```python
from build123d import *

# Parameters (mm, degrees)
BOSS_EXTRUDE4_DEPTH  = 1.5875
M3_CLEARANCE_HOLE3_D = 3
M3_CLEARANCE_HOLE1_D = 3.1
M3_CLEARANCE_HOLE4_D = 2.95
M3_CLEARANCE_HOLE2_D = 3.1
M3_CLEARANCE_HOLE5_D = 3
BOSS_EXTRUDE6_DEPTH  = 3.175
FILLET1_R            = 2
FILLET3_R            = 1


with BuildPart() as part:
    # Sketch1 → Boss-Extrude4 (new, symmetric)
    with BuildSketch(Plane(origin=(0, 0, 0), x_dir=(1, 0, 0), z_dir=(0, 1, 0))):
        with BuildLine():
            Line((-62.799553621, 32.496136604), (-73.969425011, 32.691107434))
            Line((-73.969425011, 32.691107434), (-77.053684287, 35.88495141))
            ThreePointArc((-77.053684287, 35.88495141), (-84.36642289, 10.358894189), (-83.446216027, -16.178041625))
            Line((-83.446216027, -16.178041625), (-79.680911643, -13.825218315))
            Line((-79.680911643, -13.825218315), (-69.484649137, -16.179210996))
            Line((-69.484649137, -16.179210996), (-43.894490772, -57.132025032))
            Line((-43.894490772, -57.132025032), (-43.894490772, -64.826600275))
            Line((-43.894490772, -64.826600275), (-43.094490772, -64.826600275))
            Line((-43.094490772, -64.826600275), (-34, -64.826600275))
            Line((-34, -64.826600275), (-34, -55.55))
            Line((-34, -55.55), (-34, -53.55))
            Line((-34, -53.55), (-20, -53.55))
            Line((-20, -53.55), (-19.718918331, -55.55))
            Line((-19.718918331, -55.55), (19.718918331, -55.55))
            Line((19.718918331, -55.55), (20, -53.55))
            Line((20, -53.55), (34, -53.55))
            Line((34, -53.55), (34, -55.55))
            Line((34, -55.55), (34, -64.826600275))
            Line((34, -64.826600275), (43.094490772, -64.826600275))
            Line((43.094490772, -64.826600275), (43.894490772, -64.826600275))
            Line((43.894490772, -64.826600275), (43.894490772, -57.132025032))
            Line((43.894490772, -57.132025032), (69.484649137, -16.179210996))
            Line((69.484649137, -16.179210996), (79.680911643, -13.825218315))
            Line((79.680911643, -13.825218315), (83.446216027, -16.178041625))
            ThreePointArc((83.446216027, -16.178041625), (84.610662337, -8.126242604), (85, 0))
            ThreePointArc((85, 0), (82.98964744, 18.377116688), (77.053684287, 35.88495141))
            Line((77.053684287, 35.88495141), (73.969425011, 32.691107434))
            Line((73.969425011, 32.691107434), (62.799553621, 32.496136604))
            Line((62.799553621, 32.496136604), (30.284668021, 63.895396642))
            Line((30.284668021, 63.895396642), (30.089697191, 75.065268032))
            Line((30.089697191, 75.065268032), (33.173956467, 78.259112008))
            ThreePointArc((33.173956467, 78.259112008), (0, 85), (-33.173956467, 78.259112008))
            Line((-33.173956467, 78.259112008), (-30.089697191, 75.065268032))
            Line((-30.089697191, 75.065268032), (-30.284668021, 63.895396642))
            Line((-30.284668021, 63.895396642), (-62.799553621, 32.496136604))
        make_face()
    extrude(amount=BOSS_EXTRUDE4_DEPTH, both=True)

    # M3 Clearance Hole3 (through all)
    with Locations(Plane(origin=(0, -1.5875, 0), x_dir=(-1, 0, 0), z_dir=(0, -1, 0))):
        with Locations((36.5, -50), (36.5, -38), (-36.5, -50), (-36.5, -38)):
            Hole(M3_CLEARANCE_HOLE3_D / 2)

    # M3 Clearance Hole1 (through all)
    with Locations(Plane(origin=(0, 1.5875, 0), x_dir=(1, 0, 0), z_dir=(0, 1, 0))):
        with Locations((-78.542321426, -8.49139241), (78.542321426, -8.49139241), (74.155025063, 27.240269049), (-74.155025063, 27.240269049)):
            Hole(M3_CLEARANCE_HOLE1_D / 2)

    # M3 Clearance Hole4 (through all)
    with Locations(Plane(origin=(0, -1.5875, 0), x_dir=(-1, 0, 0), z_dir=(0, -1, 0))):
        with Locations((-67.099301622, -15.278865202), (-50.141885166, -42.416404279), (-61.062544382, 30.698137949), (-38.043670771, 52.927205804), (50.141885166, -42.416404279), (67.099301622, -15.278865202), (38.043670771, 52.927205804), (61.062544382, 30.698137949)):
            Hole(M3_CLEARANCE_HOLE4_D / 2)

    # M3 Clearance Hole2 (through all)
    with Locations(Plane(origin=(0, 1.5875, 0), x_dir=(1, 0, 0), z_dir=(0, 1, 0))):
        with Locations((27, 76.497766718), (-27, 76.497766718)):
            Hole(M3_CLEARANCE_HOLE2_D / 2)

    # M3 Clearance Hole5 (through all)
    with Locations(Plane(origin=(0, 1.5875, 0), x_dir=(1, 0, 0), z_dir=(0, 1, 0))):
        with Locations((-11, -4.4), (11, -4.4), (11, -36.4), (-11, -36.4), (-11, 37.6), (11, 37.6)):
            Hole(M3_CLEARANCE_HOLE5_D / 2)

    # Sketch22 → Boss-Extrude6 (add)
    with BuildSketch(Plane(origin=(0, 1.5875, 0), x_dir=(1, 0, 0), z_dir=(0, 1, 0))):
        Polygon((65.061950694, 32.535626892), (30.245177733, 66.157793715), (30.284668021, 63.895396642), (62.799553621, 32.496136604), align=None)
        Polygon((-30.284668021, 63.895396642), (-30.245177733, 66.157793715), (-65.061950694, 32.535626892), (-62.799553621, 32.496136604), align=None)
        Polygon((43.894490772, -60.151352895), (71.689396914, -15.670204865), (69.484649137, -16.179210996), (43.894490772, -57.132025032), align=None)
        Polygon((-69.484649137, -16.179210996), (-71.689396914, -15.670204865), (-43.894490772, -60.151352895), (-43.894490772, -57.132025032), align=None)
    extrude(amount=-BOSS_EXTRUDE6_DEPTH)

    # Fillet1
    fillet1_edges = [part.edges().sort_by_distance(p)[0] for p in [
        (-30.245177733, -0.79375, -66.157793715),
        (-65.061950694, -0.79375, -32.535626892),
        (-71.689396914, 0.79375, 15.670204865),
        (-43.894490772, 0.79375, 60.151352895),
        (43.894490772, -0.79375, 60.151352895),
        (71.689396914, -0.79375, 15.670204865),
        (65.061950694, -0.79375, -32.535626892),
        (30.245177733, 0.79375, -66.157793715),
        (30.089697191, -0.79375, -75.065268032),
        (73.969425011, -0.79375, -32.691107434),
        (79.680911643, -0.79375, 13.825218315),
        (-79.680911643, -0.79375, 13.825218315),
        (-73.969425011, -0.79375, -32.691107434),
        (-30.089697191, -0.79375, -75.065268032),
    ]]
    fillet(fillet1_edges, radius=FILLET1_R)

    # Fillet3
    fillet3_edges = [part.edges().sort_by_distance(p)[0] for p in [
        (33.173956467, -0.79375, -78.259112008),
        (77.053684287, 0.79375, -35.88495141),
        (83.446216027, -0.79375, 16.178041625),
        (43.894490772, -0.79375, 64.826600275),
        (34, 0.79375, 64.826600275),
        (34, -0.79375, 53.55),
        (20, -0.79375, 53.55),
        (19.718918331, 0.79375, 55.55),
        (-19.718918331, 0.79375, 55.55),
        (-20, -0.79375, 53.55),
        (-34, -0.79375, 53.55),
        (-34, 0.79375, 64.826600275),
        (-43.894490772, -0.79375, 64.826600275),
        (-83.446216027, -0.79375, 16.178041625),
        (-77.053684287, -0.79375, -35.88495141),
        (-33.173956467, -0.79375, -78.259112008),
    ]]
    fillet(fillet3_edges, radius=FILLET3_R)


solid = part.part
```
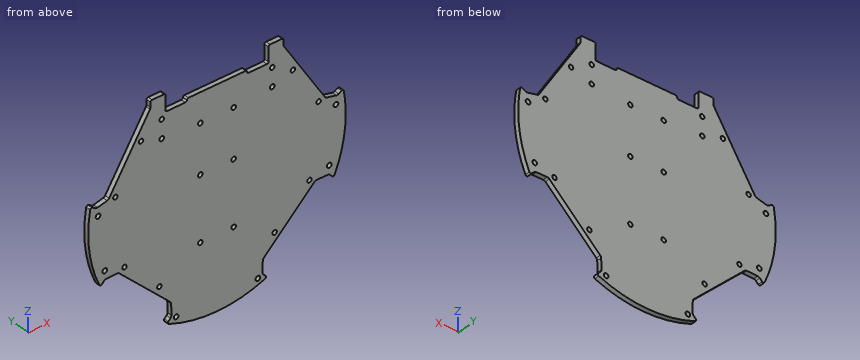
The listing builds one solid part. Answer for the finished solid, in the listing's coordinates (mm). Round coordinates to 2 decimals unless told otherwise and drop trailing zeros. Loops run counter-clockwise (first coordinate to the right, second up) from the corner with the lowest first, then second, coordinate; pieces in that order, holes last.
Q1. Section B-B, the plane y = 0.4 is taken. Count the separate pieces of the cut face and the enclosed holes in it, then the cut area to 3 significant figures.
Q2. Section A-A, the plane z = 27 is taken. Determine the outline of the cut face in (x, y).
Q3. Given pin 1 Ø2.5 at (x, z) = (-50.14, 42.42) entering from -Y; pin 2 Ø1.5 at (x, y) = (-11.5, 1) entering from +Z; pin 3 Ø0.9 at (y, z) = (-0.5, 62) entering from -X; pin 4 Ø4.5 at (x, z) = (67.1, 15.28) entering from +Y, each flat-ended and moving along its own axis, determine where each tip first touches the part or whether it passes through.
Q4. Find the intervals of material crossed by line 1 (X direction, y = -1.1, z = -27.5); line 2 (X direction, y = 0.95, z = -38); line 3 (Z direction, x = 36.5, y = 0.55), in increasing order.
Q5. Section C-C, the plane z = -61.5 is taken. Determine the outline of the cut face in (x, y), then the cut area to 3 significant figures.
Completed:
1. separate pieces: 1
1. enclosed holes: 24
1. area: 17,000 mm2
2. outline: (-64.61, -1.59) - (64.61, -1.59) - (64.61, 1.59) - (-64.61, 1.59) - close
3. pin 1: passes through
3. pin 2: stops at z = 55.55
3. pin 3: stops at x = -43.89
3. pin 4: stops at y = 1.59
4. line 1: x = -80.43 to -75.68, -72.63 to 72.63, 75.68 to 80.43
4. line 2: x = -59.4 to -12.45, -9.55 to 9.55, 12.45 to 59.4
4. line 3: z = -60.12 to 36.5, 39.5 to 48.5, 51.5 to 64.83
5. outline: (-35.07, -1.59) - (35.07, -1.59) - (35.07, 1.59) - (-35.07, 1.59) - close
5. area: 223 mm2
